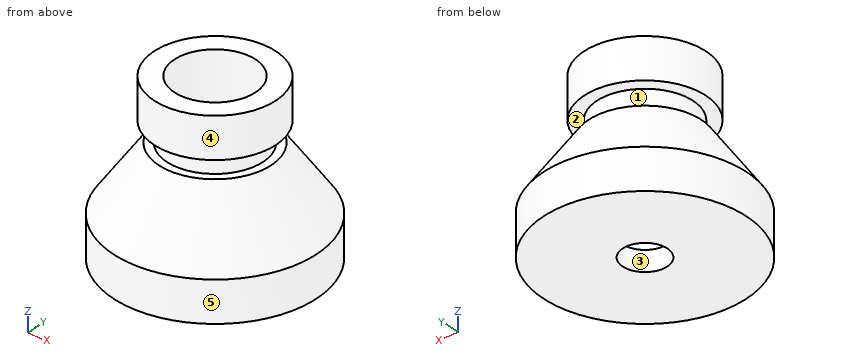
```python
from build123d import *

# Parameters (mm, degrees)
F2_R     = 5.5
F3_DEPTH = 25


with BuildPart() as f1:
    # F0 (on Front) → F1 (revolve)
    with BuildSketch(Plane.XZ):
        Polygon((-25, 0), (0, 0), (0, 5), (-10, 5), (-10, 40.923497), (-15, 40.923497), (-15, 30.923497), (-11.850247, 30.923497), (-11.850247, 25.923497), (-13.850247, 25.923497), (-25, 10), align=None)
    revolve(axis=Axis((0, 0, 25), (0, 0, 1)))

    # F2 (on face) → F3 (cut)
    with BuildSketch(Plane(origin=(0, 0, 0), x_dir=(1, 0, 0), z_dir=(0, 0, -1))):
        Circle(F2_R)
    extrude(amount=-F3_DEPTH, mode=Mode.SUBTRACT)


solid = f1.part
```
For this review, take the finished solid that the model builds, in its own axes (mm). Face numbers are marked on the shaded views. A direction names the side the tool comes from. Coordinates: 2 decimals unless noted, no trailing zeros. Write each loop counter-clockwise with the first axis right and the second up, starting at its lowest first coordinate (ties: lowest second). Pieces come first, ordered by that corner, then holes. Notation, with made-up numbers: (66.5, 19.25) -> (73.5, 19.25) arc R21 ccw to (73.5, 31.25) -> close; hole circle Ø5 at (2, -24). An arc over 180 degrees is marked (long way). Put each result on its own line as item: value.
Q1. Take a section at D-D, the plane z = 9. State the section outline as (x, y) points.
From the geometry:
outline: circle Ø50 at (0, 0); hole circle Ø20 at (0, 0)
Q2. Clearance check with flat-ended pins moving along their axes: pin 1 Ø12.5 at (x, y) = (0, 0) entering from +Z; pin 2 Ø5 at (x, z) = (9.5, 22) entering from +Y; pin 3 Ø6 at (x, z) = (-10.5, 11) entering from +Y. State where each tip first meets the part, or that it passes through.
From the geometry:
pin 1: stops at z = 5
pin 2: stops at y = 16.13
pin 3: stops at y = 23.79
Q3. Take a section at C-C, the plane z = 36.5. State the section outline as (x, y) points, then the cut area to 3 significant figures.
From the geometry:
outline: circle Ø30 at (0, 0); hole circle Ø20 at (0, 0)
area: 393 mm2
Q4. Wall thickness on L1, parallel to Y at x = 0, z = 2.65; L2, parallel to X at y = 0, z = 26: over which ranges is each line inside the solid? List them lowest first.
From the geometry:
L1: y = -25 to -5.5, 5.5 to 25
L2: x = -11.85 to -10, 10 to 11.85
Q5. The part is to be moulded in two halves that separate along Y. For the marked faces 1, 2 and 3, say which applies: +Y half, -Y half, draft (parallel to the pull), parting line (faces both ways), or undercut.
From the geometry:
face 1: parting line
face 2: draft
face 3: undercut
Q6. Take a section at A-A, the plane x = 0. State the section outline as (y, z) points.
From the geometry:
outline: (-25, 0) -> (-5.5, 0) -> (-5.5, 5) -> (-10, 5) -> (-10, 40.92) -> (-15, 40.92) -> (-15, 30.92) -> (-11.85, 30.92) -> (-11.85, 25.92) -> (-13.85, 25.92) -> (-25, 10) -> close; (5.5, 0) -> (25, 0) -> (25, 10) -> (13.85, 25.92) -> (11.85, 25.92) -> (11.85, 30.92) -> (15, 30.92) -> (15, 40.92) -> (10, 40.92) -> (10, 5) -> (5.5, 5) -> close
Q7. Tool access review of the marked faces 4 and 5: name each direction out of +Z, -Z, +X, -X, +Y, -Y from which nothing blocks a thin tool from reaching the whole face with its end or side.
From the geometry:
face 4: +Z
face 5: +Z, -Z
